from build123d import *

# Parameters (mm, degrees)
SKETCH1_R           = 0.75
SKETCH1_R_2         = 0.5
BOSS_EXTRUDE1_DEPTH = 4
SKETCH2_W           = 16.2
SKETCH2_H           = 9.205
CUT_EXTRUDE1_DEPTH  = 2


with BuildPart() as part:
    # Sketch1 → Boss-Extrude1 (new body)
    with BuildSketch(Plane.XY):
        with BuildLine():
            Line((12.2, 4), (16.2, 4))
            Line((16.2, 4), (16.2, 2))
            ThreePointArc((16.2, 2), (15.614213562, 0.585786438), (14.2, 0))
            Line((14.2, 0), (2, 0))
            ThreePointArc((2, 0), (0.585786438, 0.585786438), (0, 2))
            Line((0, 2), (0, 4))
            Line((0, 4), (4, 4))
            Line((4, 4), (4, 6))
            Line((4, 6), (0, 6))
            Line((0, 6), (0, 9.205))
            ThreePointArc((0, 9.205), (1.464466094, 12.740533906), (5, 14.205))
            Line((5, 14.205), (11.2, 14.205))
            ThreePointArc((11.2, 14.205), (14.735533906, 12.740533906), (16.2, 9.205))
            Line((16.2, 9.205), (16.2, 6))
            Line((16.2, 6), (12.2, 6))
            Line((12.2, 6), (12.2, 4))
        make_face()
        with Locations(Location((13.45, 2, 0), (0, 0, 180))):
            Circle(SKETCH1_R, mode=Mode.SUBTRACT)
        with Locations(Location((13.2, 11.205, 0), (0, 0, 180))):
            Circle(SKETCH1_R_2, mode=Mode.SUBTRACT)
        with Locations(Location((10.2, 7.75, 0), (0, 0, 180))):
            Circle(SKETCH1_R, mode=Mode.SUBTRACT)
        with Locations((6, 7.75)):
            Circle(SKETCH1_R, mode=Mode.SUBTRACT)
        with Locations((3, 11.205)):
            Circle(SKETCH1_R_2, mode=Mode.SUBTRACT)
        with Locations((2.75, 2)):
            Circle(SKETCH1_R, mode=Mode.SUBTRACT)
    extrude(amount=BOSS_EXTRUDE1_DEPTH)

    # Sketch2 → Cut-Extrude1 (cut)
    with BuildSketch(Plane(origin=(0, 0, 0), x_dir=(-1, 0, 0), z_dir=(0, 0, -1))):
        with Locations((-8.1, 4.6025)):
            Rectangle(SKETCH2_W, SKETCH2_H)
    extrude(amount=-CUT_EXTRUDE1_DEPTH, mode=Mode.SUBTRACT)


solid = part.part
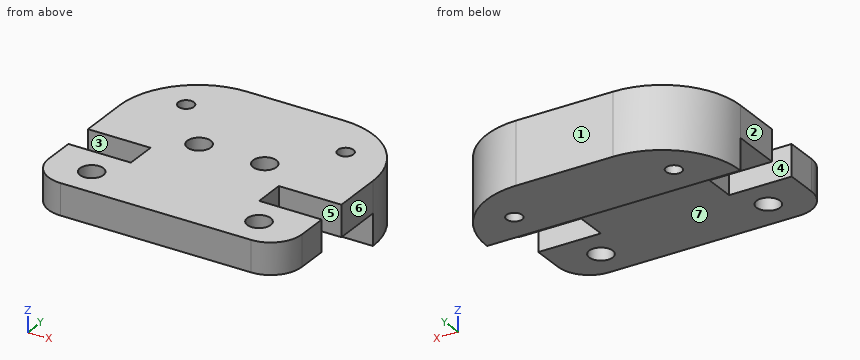
Geometry: final body of the model. Coordinates: model frame, mm. Face numbers are marked on the shaded views. A direction names the side the tool comes from. Round coordinates to 2 decimals unless told otherwise and drop trailing zeros. Loops run counter-clockwise (first coordinate to the right, second up) from the corner with the lowest first, then second, coordinate; pieces in that order, holes last. Notation, with made-up numbers: (21.5, 72.25) -> (62.5, 72.25) arc R25 cw to (62.5, 93.25) -> close; hole circle Ø10 at (-0.5, 50). An arc over 180 degrees is marked (long way). One line per question, with ' | ' between items. Start each with the question number.
1. Section B-B on y = 7.75. Output: boundary loops of the cut face in (x, z), and give its area (3 significant figures).
2. Mould query, pull axis Y, two halves, no side actions, for the marked faces 1, 2 and 3. Classes: pulls with the +Y half, pulls with the -Y half, needs draft (parallel to the pull), parting line crosses it, or undercut.
3. Section A-A on x = 6. Output: boundary loops of the cut face in (y, z) (3 decimals), and give its area (3 significant figures).
4. Section D-D on x = 3. Output: boundary loops of the cut face in (y, z) (3 decimals), and give its area (3 significant figures).
5. Contact query for flat-ended pins moving along their axis: pin 1 (2 mm diameter, centred on x = 10.2, y = 7.75, fed in from -Z); pin 2 (1 mm diameter, centred on x = 13, z = 2.5, fed in from +Y); pin 3 (0.6 mm diameter, centred on x = 1.5, z = 3, fed in from -Y); pin 4 (0.9 mm diameter, centred on x = 13.45, y = 2, fed in from +Z). Output: stop coordinate, or through.
6. Section C-C on z = 0.45. Output: boundary loops of the cut face in (x, y) (3 decimals), and give its area (3 significant figures).
7. Line query: line 1 along X through (y, z) = (2, 2.5); line 2 along Y through (x, z) = (6, 3.55) (3 decimals); line 3 along Y through (x, z) = (4.75, 2.85). Output: solid intervals per line, ascending. Write a range as [from, to].
8. Set-up query: the marked faces 4, 5, 6 and 7. Return all of +Z, -Z, +X, -X, +Y, -Y with unobstructed straight access to the full face (end or side cutting, diameter ignored); none if empty.
Returned:
1) outline: (0, 2) -> (5.25, 2) -> (5.25, 4) -> (0, 4) -> close; (6.75, 2) -> (9.45, 2) -> (9.45, 4) -> (6.75, 4) -> close; (10.95, 2) -> (16.2, 2) -> (16.2, 4) -> (10.95, 4) -> close | area: 26.4 mm2
2) face 1: pulls with the +Y half | face 2: needs draft | face 3: undercut
3) outline: (0, 2) -> (7, 2) -> (7, 4) -> (0, 4) -> close; (8.5, 2) -> (9.205, 2) -> (9.205, 0) -> (14.205, 0) -> (14.205, 4) -> (8.5, 4) -> close | area: 35.4 mm2
4) outline: (0, 2) -> (1.293, 2) -> (1.293, 4) -> (0, 4) -> close; (2.707, 2) -> (4, 2) -> (4, 4) -> (2.707, 4) -> close; (6, 2) -> (9.205, 2) -> (9.205, 0) -> (10.705, 0) -> (10.705, 4) -> (6, 4) -> close; (11.705, 0) -> (13.788, 0) -> (13.788, 4) -> (11.705, 4) -> close | area: 25.9 mm2
5) pin 1: stops at z = 2 | pin 2: stops at y = 14.03 | pin 3: stops at y = 0.01 | pin 4: passes through
6) outline: (0, 9.205) -> (16.2, 9.205) arc R5 ccw to (11.2, 14.205) -> (5, 14.205) arc R5 ccw to start; hole circle Ø1 at (3, 11.205); hole circle Ø1 at (13.2, 11.205) | area: 68.7 mm2
7) line 1: x = [0, 2], [3.5, 12.7], [14.2, 16.2] | line 2: y = [0, 7], [8.5, 14.205] | line 3: y = [0, 14.2]
8) face 4: +Z, -Z, -X | face 5: +Z, -Z, +X | face 6: +Z, -Z, +X, +Y, -Y | face 7: -Z, +X, -X, -Y
